Drawing for the job (mm, zero at the part's lowest x, y, z). Give positions to 0.01 mm unless a question says otherwise; leave off trailing zeros. Write each loop counter-clockwise with the first axis right and the second up, starting at its lowest first coordinate (ties: lowest second). Pieces come first, ordered by that corner, then holes. Notation, with made-up numbers: M -38.5,36.25 L -16.5,36.25 A11 cw -16.5,44.25 Z; hole C 54.25,83 d5. An arc over 180 degrees is marked long. Write item = value, one per line. Start each with the question number.
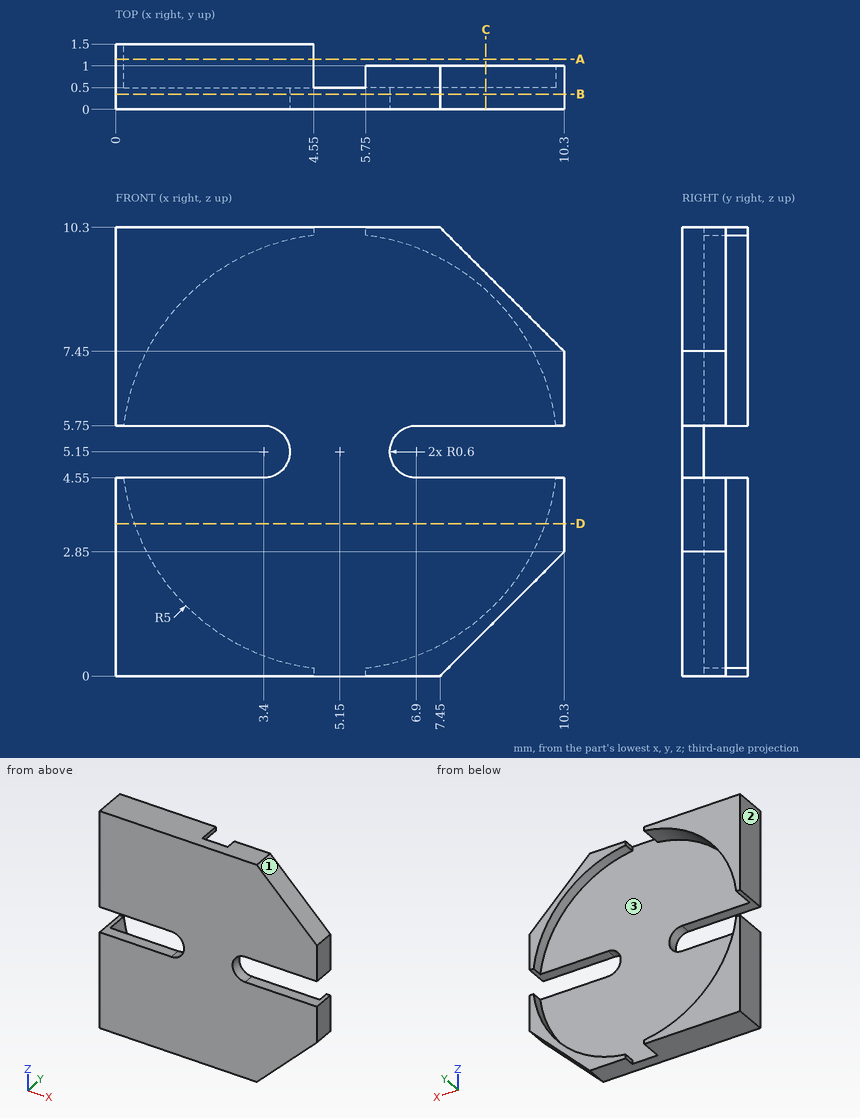
Q1. Drop flat-ended pins along their axis: P1, Ø1, axis at x = 6.5, z = 6.5, coming from the +Y side; P2, Ø2.5, axis at x = 9, z = 2, coming from the +Y side. Give the stop position or say it passes through.
Q2. Slice it at D-D (z = 3.5). Give the cut face in (x, y).
Q3. Two-plate mould, pull along X, no slides. Class the marked faces 1, 2 and 3: +X half, -X half, draft (parallel to the pull), parting line (faces both ways), or undercut.
Q4. Slice it at B-B (y = 0.35). Give the cut face in (x, z), and give its area (3 significant figures).
Q5. Probe line 1 along Z through (x, y) = (0.75, 0.15); line 2 along Y through (x, z) = (8.25, 7.5); line 3 along Z through (x, y) = (6, 0.9). List the from-to ranges inside material, lowest first.
Q6. Slice it at A-A (y = 1.15). Give the cut face in (x, z).
Q7. Slice it at C-C (x = 8.5). Give the cut face in (y, z).
Working result:
q1.P1 = 0.5
q1.P2 = 1
q2.outline = M 0,0 L 10.3,0 L 10.3,1 L 9.87,1 L 9.87,0.5 L 0.43,0.5 L 0.43,1.5 L 0,1.5 Z
q3.face_1 = +X half
q3.face_2 = -X half
q3.face_3 = undercut
q4.outline = M 0,0 L 7.45,0 L 10.3,2.85 L 10.3,4.55 L 6.9,4.55 A0.6 cw 6.9,5.75 L 10.3,5.75 L 10.3,7.45 L 7.45,10.3 L 0,10.3 L 0,5.75 L 3.4,5.75 A0.6 cw 3.4,4.55 L 0,4.55 Z
q4.area = 88.7 mm2
q5.line_1 = 0 to 4.55, 5.75 to 10.3
q5.line_2 = 0 to 0.5
q5.line_3 = 0 to 0.22, 10.08 to 10.3
q6.outline = M 0,0 L 4.55,0 L 4.55,0.19 A5 cw 0.19,4.55 L 0,4.55 Z; M 0,5.75 L 0.19,5.75 A5 cw 4.55,10.11 L 4.55,10.3 L 0,10.3 Z
q7.outline = M 0,1.05 L 1,1.05 L 1,1.44 L 0.5,1.44 L 0.5,4.55 L 0,4.55 Z; M 0,5.75 L 0.5,5.75 L 0.5,8.86 L 1,8.86 L 1,9.25 L 0,9.25 Z
